Verification items for the finished model (mm, model axes). A direction names the side the tool comes from. Round coordinates to 2 decimals unless told otherwise and drop trailing zeros. Write each loop counter-clockwise with the first axis right and the second up, starting at its lowest first coordinate (ties: lowest second). Pieces come first, ordered by that corner, then holes. Notation, with made-up numbers: M -24,82 L 33,82 A30 ccw 33,105 Z; hole C 51.25,47 d7. An arc over 180 degrees is marked long. One line per question, with ' | ' between items.
from build123d import *

# Parameters (mm, degrees)
SKETCH1_R               = 23.5
BOSS_EXTRUDE1_DEPTH     = 40
CUT_EXTRUDE1_DEPTH      = 102.443199391
CUT_EXTRUDE1_DEPTH_BACK = 102.443199391
SKETCH2_R               = 7.5


with BuildPart() as part:
    # Sketch1 → Boss-Extrude1 (new body)
    with BuildSketch(Plane.XY):
        with BuildLine():
            Line((-30, 0), (-30, -45.991596264))
            Line((-30, -45.991596264), (-54, -45.991596264))
            Line((-54, -45.991596264), (-54, -56.568744975))
            Line((-54, -56.568744975), (54, -56.568744975))
            Line((54, -56.568744975), (54, -45.991596264))
            Line((54, -45.991596264), (30, -45.991596264))
            Line((30, -45.991596264), (30, 0))
            ThreePointArc((30, 0), (0, 30), (-30, 0))
        make_face()
        Circle(SKETCH1_R, mode=Mode.SUBTRACT)
    extrude(amount=BOSS_EXTRUDE1_DEPTH)

    # Sketch2 → Cut-Extrude1 (cut, two sides: drawn at the far end of the back side and taken through both)
    with BuildSketch(Plane(origin=(0, -45.991596264, 0), x_dir=(1, 0, 0), z_dir=(0, 1, 0)).offset(-CUT_EXTRUDE1_DEPTH_BACK)):
        with Locations(Location((42, -20, 0), (0, 0, 180))):
            Circle(SKETCH2_R)
        with Locations(Location((-42, -20, 0), (0, 0, 90))):
            Circle(SKETCH2_R)
    extrude(amount=CUT_EXTRUDE1_DEPTH + CUT_EXTRUDE1_DEPTH_BACK, mode=Mode.SUBTRACT)


solid = part.part
1. Section check B-B, the plane z = 14. Record the cut outline in (x, y), then the cut area to 3 significant figures.
Results:
outline: M -54,-56.57 L -46.5,-56.57 L -46.5,-45.99 L -54,-45.99 Z; M -37.5,-56.57 L 37.5,-56.57 L 37.5,-45.99 L 30,-45.99 L 30,0 A30 ccw -30,0 L -30,-45.99 L -37.5,-45.99 Z; M 46.5,-56.57 L 54,-56.57 L 54,-45.99 L 46.5,-45.99 Z; hole C 0,0 d47 | area: 3,390 mm2
2. Mould release check, pull along X, two halves, no side actions. Record for faces 4 (the face through (37.968, -51.354, 26.324)), 5 (the face through (-34.68, -51.35, 21.63)), 6 (the face through (54, -51, 20)), 7 (the face through (0.66, 29.993, 19.72)): pulls with the +X half, pulls with the -X half, needs draft (parallel to the pull), parting line crosses it, or undercut.
Results:
face 4: undercut | face 5: undercut | face 6: pulls with the +X half | face 7: parting line crosses it
3. Section check A-A, the plane x = 0. Record the cut outline in (y, z).
Results:
outline: M -56.57,0 L -23.5,0 L -23.5,40 L -56.57,40 Z; M 23.5,0 L 30,0 L 30,40 L 23.5,40 Z
4. Section check D-D, the plane z = 34. Record the cut outline in (x, y).
Results:
outline: M -54,-56.57 L 54,-56.57 L 54,-45.99 L 30,-45.99 L 30,0 A30 ccw -30,0 L -30,-45.99 L -54,-45.99 Z; hole C 0,0 d47
5. Section check C-C, the plane y = 19.5. Record the cut outline in (x, z).
Results:
outline: M -22.8,0 L -13.11,0 L -13.11,40 L -22.8,40 Z; M 13.11,0 L 22.8,0 L 22.8,40 L 13.11,40 Z
6. Go/stop test with flat-tipped pins: P1, Ø5, axis at x = 2, z = 15.5, coming from the +Y side; P2, Ø12, axis at x = 37.5, z = 11, coming from the +Y side; P3, Ø3, axis at x = -11, z = 27, coming from the +Y side. Record where each tip stops, or that it passes through.
Results:
P1: stops at y = 30 | P2: stops at y = -45.99 | P3: stops at y = 28.46
7. Thickness scan on line 1 (X direction, y = -54, z = 20); line 2 (Z direction, x = 42, y = -48.75); line 3 (Y direction, x = 0, z = 22). Record the ranges inside material, lowest first.
Results:
line 1: x = -54 to -49.5, -34.5 to 34.5, 49.5 to 54 | line 2: z = 0 to 12.5, 27.5 to 40 | line 3: y = -56.57 to -23.5, 23.5 to 30
8. Tool access check on faces 1 (the face through (34, -45.992, 20)), 2 (the face through (-30, -23, 20)), 3 (the face through (-1, -32, 40)). Record the directions out of +Z, -Z, +X, -X, +Y, -Y that give a thin tool (end or side, any length) a straight path to the whole face; none if there is none.
Results:
face 1: +Z, -Z, +X, +Y | face 2: +Z, -Z, -X, +Y | face 3: +Z, +X, -X, +Y, -Y
